Could you check a few things on this model? Use its own coordinates, in mm. Face numbers are marked on the shaded views. A direction names the side the tool comes from. Give positions to 0.01 mm unless a question says otherwise; leave off trailing zeros. Write each loop counter-clockwise with the first axis right and the second up, starting at its lowest first coordinate (ties: lowest second). Pieces come first, ordered by that corner, then holes. Notation, with made-up numbers: M 27.5,63 L 80.5,63 A26 cw 80.5,77 Z; hole C 3.25,39.5 d9. An arc over 180 degrees is marked long. Use one line per item in the form item = value.
from build123d import *

# Parameters (mm, degrees)
SKETCH1_R           = 1.65
BOSS_EXTRUDE1_DEPTH = 1


with BuildPart() as part:
    # Sketch1 → Boss-Extrude1 (new body, symmetric)
    with BuildSketch(Plane.XY):
        with BuildLine():
            Line((-10, 15), (-10, -15))
            Line((-10, -15), (10, -15))
            Line((10, -15), (10, -5))
            Line((10, -5), (1.65, -5))
            ThreePointArc((1.65, -5), (-1.166726189, -6.166726189), (0, -3.35))
            Line((0, -3.35), (0, 15))
            Line((0, 15), (-10, 15))
        make_face()
        with Locations((-5, 10)):
            Circle(SKETCH1_R, mode=Mode.SUBTRACT)
        with Locations((-5, 0)):
            Circle(SKETCH1_R, mode=Mode.SUBTRACT)
        with Locations((5, -10)):
            Circle(SKETCH1_R, mode=Mode.SUBTRACT)
        with Locations((-5, -10)):
            Circle(SKETCH1_R, mode=Mode.SUBTRACT)
    extrude(amount=BOSS_EXTRUDE1_DEPTH, both=True)


solid = part.part
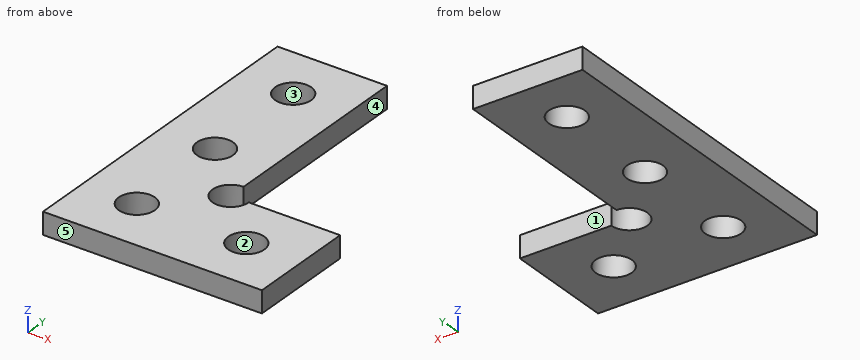
1) Thinking about a two-plate mould opening in X: for the marked faces 3, 4 and 5, which applies, released by +X, released by -X, zero draft, split by the parting line, or undercut?
Checked values:
face_3 = undercut
face_4 = released by +X
face_5 = zero draft
2) I want a section at D-D, the plane x = 5. Please give me the cut outline in (y, z), plus the area to 3 significant figures.
Checked values:
outline = M -15,-1 L -11.65,-1 L -11.65,1 L -15,1 Z; M -8.35,-1 L -5,-1 L -5,1 L -8.35,1 Z
area = 13.4 mm2
3) I want a section at C-C, the plane x = -5. Please give me the cut outline in (y, z).
Checked values:
outline = M -15,-1 L -11.65,-1 L -11.65,1 L -15,1 Z; M -8.35,-1 L -1.65,-1 L -1.65,1 L -8.35,1 Z; M 1.65,-1 L 8.35,-1 L 8.35,1 L 1.65,1 Z; M 11.65,-1 L 15,-1 L 15,1 L 11.65,1 Z
4) I want a section at B-B, the plane z = -0.6. Please give me the cut outline in (x, y).
Checked values:
outline = M -10,-15 L 10,-15 L 10,-5 L 1.65,-5 A1.65 cw long 0,-3.35 L 0,15 L -10,15 Z; hole C -5,-10 d3.3; hole C -5,0 d3.3; hole C -5,10 d3.3; hole C 5,-10 d3.3
5) For pin 1 Ø3 at (x, y) = (5, -10) entering from -Z; pin 2 Ø0.6 at (x, z) = (4.5, 0) entering from +Y; pin 3 Ø12 at (x, y) = (-4.5, 8.5) entering from -Z, each with a flat end and sliding along its axis, tell me the tip position at first contact or that it passes through.
Checked values:
pin_1 = through
pin_2 = -5
pin_3 = -1
6) For the marked faces 1 and 2, which set-ups out of +Z, -Z, +X, -X, +Y, -Y let a thin tool reach every point of the face, with its end or its side?
Checked values:
face_1 = +Z, -Z, +X, +Y
face_2 = +Z, -Z
7) If I drill on L1, parallel to Y at x = -5, z = 0.35; L2, parallel to Y at x = -5.75, z = -0.7; L3, parallel to X at y = 2.75, z = 0.8, over which ranges is the centre line in solid material (lowest first)?
Checked values:
L1 = -15 to -11.65, -8.35 to -1.65, 1.65 to 8.35, 11.65 to 15
L2 = -15 to -11.47, -8.53 to -1.47, 1.47 to 8.53, 11.47 to 15
L3 = -10 to 0
8) I want a section at A-A, the plane y = -10. Please give me the cut outline in (x, z), plus the area to 3 significant figures.
Checked values:
outline = M -10,-1 L -6.65,-1 L -6.65,1 L -10,1 Z; M -3.35,-1 L 3.35,-1 L 3.35,1 L -3.35,1 Z; M 6.65,-1 L 10,-1 L 10,1 L 6.65,1 Z
area = 26.8 mm2
